from build123d import *

# Parameters (mm, degrees)
F0_W     = 31.75
F0_H     = 31.75
F0_R     = 3.175
F1_DEPTH = 6.35
F0_W_2   = 6.35
F2_DEPTH = 25.4
F3_R     = 3.175
F4_DEPTH = 25.4


with BuildPart() as f1:
    # F0 (on Top) → F1 (new body)
    with BuildSketch(Plane.XY):
        Rectangle(F0_W, F0_H)
        with Locations((7.9375, -7.9375)):
            Circle(F0_R, mode=Mode.SUBTRACT)
        with Locations((7.9375, 7.9375)):
            Circle(F0_R, mode=Mode.SUBTRACT)
    extrude(amount=F1_DEPTH)

    # F0 (on Top) → F2 (join)
    with BuildSketch(Plane.XY):
        with Locations((-19.05, 0)):
            Rectangle(F0_W_2, F0_H)
    extrude(amount=F2_DEPTH)

    # F3 (on face) → F4 (cut)
    with BuildSketch(Plane.YZ.offset(-15.875)):
        with Locations((-7.9375, 19.4)):
            Circle(F3_R)
        with Locations((7.9375, 19.4)):
            Circle(F3_R)
    extrude(amount=-F4_DEPTH, mode=Mode.SUBTRACT)


solid = f1.part
Geometry: final body of the model. Coordinates: model frame, mm. A direction names the side the tool comes from. Round coordinates to 2 decimals unless told otherwise and drop trailing zeros. Order: outer loops, then holes, each group sorted by start corner. A loop starts at its lowest first (then second) coordinate and runs counter-clockwise, first axis right, second up.
Q1. Section A-A, the plane z = 19.4. Output: boundary loops of the cut face in (x, y) (1 decimal).
Result sheet:
outline: (-22.2, -15.9) - (-15.9, -15.9) - (-15.9, -11.1) - (-22.2, -11.1) - close; (-22.2, -4.8) - (-15.9, -4.8) - (-15.9, 4.8) - (-22.2, 4.8) - close; (-22.2, 11.1) - (-15.9, 11.1) - (-15.9, 15.9) - (-22.2, 15.9) - close
Q2. Section C-C, the plane x = 10.5. Output: boundary loops of the cut face in (y, z) (3 decimals).
Result sheet:
outline: (-15.875, 0) - (-9.812, 0) - (-9.812, 6.35) - (-15.875, 6.35) - close; (-6.063, 0) - (6.063, 0) - (6.063, 6.35) - (-6.063, 6.35) - close; (9.812, 0) - (15.875, 0) - (15.875, 6.35) - (9.812, 6.35) - close
Q3. Section B-B, the plane y = 10.5. Output: boundary loops of the cut face in (x, z) (3 decimals).
Result sheet:
outline: (-22.225, 0) - (6.063, 0) - (6.063, 6.35) - (-15.875, 6.35) - (-15.875, 17.525) - (-22.225, 17.525) - close; (-22.225, 21.275) - (-15.875, 21.275) - (-15.875, 25.4) - (-22.225, 25.4) - close; (9.812, 0) - (15.875, 0) - (15.875, 6.35) - (9.812, 6.35) - close
Q4. Section D-D, the plane x = -17.5. Give the number of separate pieces and of enclosed holes in the cut face, and give its area (3 significant figures).
Result sheet:
separate pieces: 1
enclosed holes: 2
area: 743 mm2
Q5. Pin query (flat end, axial travel): pin 1 (12 mm diameter, centred on y = -7.5, z = 17, fed in from +X) (3 decimals); pin 2 (5 mm diameter, centred on x = -6.5, z = 8, fed in from +Y) (3 decimals); pin 3 (8.5 mm diameter, centred on x = 7.94, y = 7.94, fed in from +Z). Return the tip coordinate at first contact, or that it passes through.
Result sheet:
pin 1: stops at x = -15.875
pin 2: stops at y = 15.875
pin 3: stops at z = 6.35
Q6. Material intervals for probe 1 along Z at (x, y) = (7.5, 3.5); probe 2 along Z at (x, y) = (-16, -9.5); probe 3 along X at (y, z) = (12, 14) (3 decimals), sorted ascending.
Result sheet:
probe 1: z = 0 to 6.35
probe 2: z = 0 to 16.64, 22.16 to 25.4
probe 3: x = -22.225 to -15.875
Q7. Access query for faces 5 (the face through (-15.875, 0, 16)), 6 (the face through (-19.006, 7.524, 22.548)). Directions: +Z, -Z, +X, -X, +Y, -Y. A direction counts if a zero-diameter tool reaches every point of the face in a straight line with its end or side. Return the directions, or none.
Result sheet:
face 5: +Z, +X, +Y, -Y
face 6: +X, -X
Q8. Mould query, pull axis Y, two halves, no side actions, for faces 1 (the face through (15.875, 0, 3)), 2 (the face through (-19.01, -8.35, 22.55)), 3 (the face through (9.403, -10.754, 3.131)), 4 (the face through (-12, -15.875, 4)). Classes: released by +Y, released by -Y, zero draft, split by the parting line, or undercut.
Result sheet:
face 1: zero draft
face 2: undercut
face 3: undercut
face 4: released by -Y
